The drawing under review shows one solid part. Ordinate dimensions are in mm from its lowest x, y, z. Give positions to 0.01 mm unless a question says otherwise; leave off trailing zeros. Write each loop counter-clockwise with the first axis right and the second up, starting at its lowest first coordinate (ties: lowest second). Pieces come first, ordered by that corner, then holes. Notation, with made-up numbers: (50.25, 13.25) -> (82.25, 13.25) arc R19 cw to (82.25, 21.25) -> close; hole circle Ø11 at (33.25, 85). An arc over 180 degrees is marked (long way). Use CSV: the item, a comma, the result in double quotes.
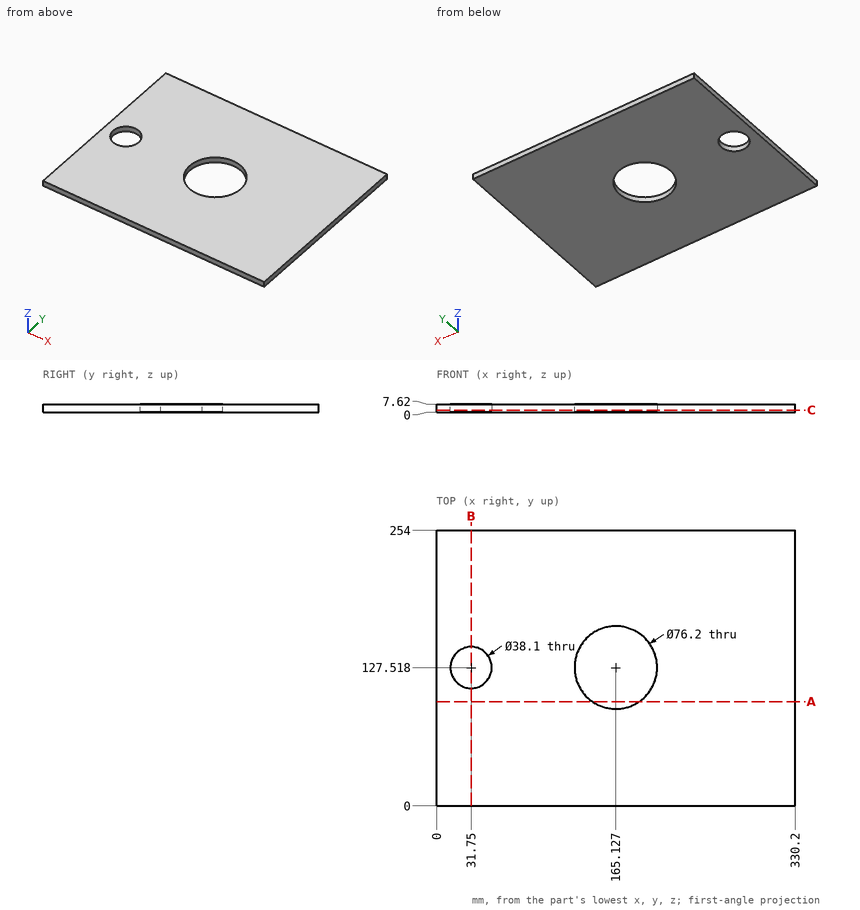
(1) Take a section at A-A (y = 96). Write out the cut boundary in (x, z), then the cut area to 3 significant figures.
Established:
outline,"(0, 0) -> (143.72, 0) -> (143.72, 7.62) -> (0, 7.62) -> close; (186.53, 0) -> (330.2, 0) -> (330.2, 7.62) -> (186.53, 7.62) -> close"
area,"2,190 mm2"
(2) Take a section at C-C (z = 2). Write out the cut boundary in (x, y), then the cut area to 3 significant figures.
Established:
outline,"(0, 0) -> (330.2, 0) -> (330.2, 254) -> (0, 254) -> close; hole circle Ø38.1 at (31.75, 127.52); hole circle Ø76.2 at (165.13, 127.52)"
area,"78,200 mm2"
(3) Take a section at B-B (x = 31.75). Write out the cut boundary in (y, z).
Established:
outline,"(0, 0) -> (108.47, 0) -> (108.47, 7.62) -> (0, 7.62) -> close; (146.57, 0) -> (254, 0) -> (254, 7.62) -> (146.57, 7.62) -> close"
(4) For line 1 along Y through (x, z) = (31.75, 4.5); line 2 along X through (y, z) = (115, 5); line 3 along Y through (x, z) = (21, 2) (1 decimal), list the stretches that pass through material, from the lowest coordinate up. Write a range as [from, to].
Established:
line 1,"y = [0, 108.47], [146.57, 254]"
line 2,"x = [0, 17.39], [46.11, 129.14], [201.11, 330.2]"
line 3,"y = [0, 111.8], [143.2, 254]"
